Input: dimensioned drawing with shaded views. Units: mm. Origin: part minimum x, y, z. Give positions to 0.01 mm unless a question says otherwise; leave off trailing zeros. Write each loop counter-clockwise with the first axis right and the second up, starting at its lowest first coordinate (ties: lowest second). Pieces come first, ordered by that corner, then holes. Notation, with made-up numbers: (85, 56) -> (117, 56) arc R22 cw to (117, 68) -> close; hole circle Ø5 at (-36.75, 42). An arc over 180 degrees is marked (long way). Answer in a Markdown table with one row per item. Add a question column.
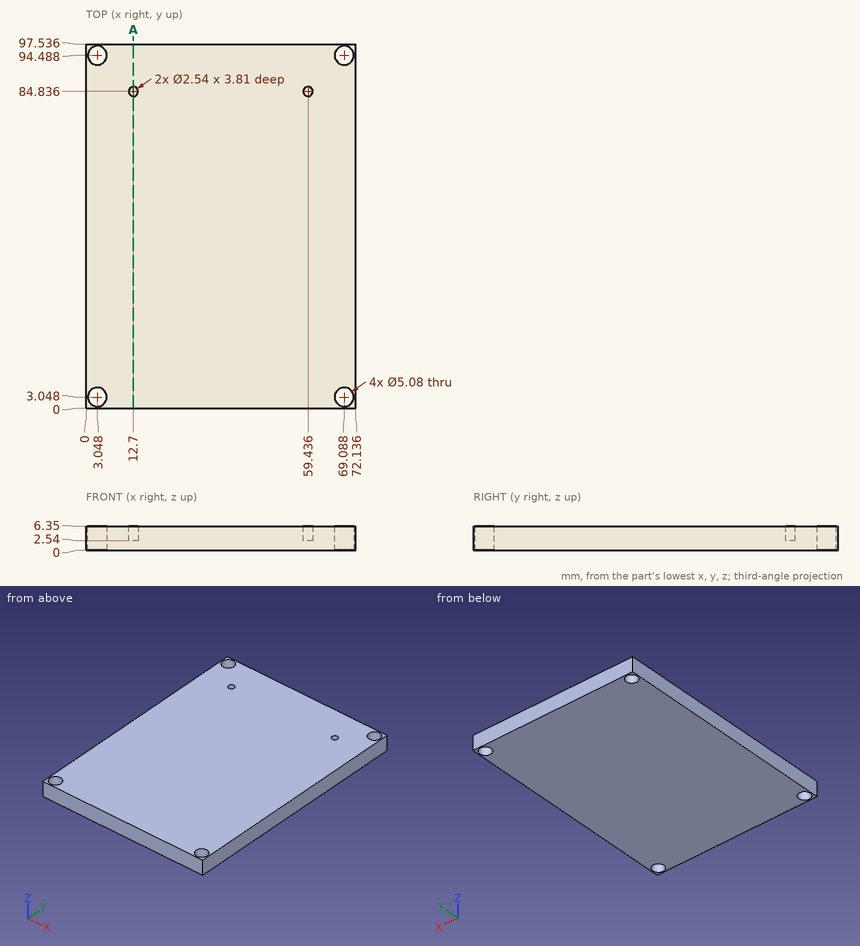
Q1. Line query: probe 1 along Y at (x, z) = (69, 5.25); probe 2 along X at (y, z) = (92.5, 5); probe 3 along Y at (x, z) = (12.7, 4.85). Output: solid intervals per line, ascending. Write a range as from..to.
Q2. Section A-A on x = 12.7. Return loops of the section in (y, z), and give its area (3 significant figures).
Q3. Contact query for flat-ended pins moving along their axis: pin 1 Ø3 at (x, y) = (3.048, 3.048) entering from -Z; pin 2 Ø0.8 at (x, y) = (59, 84.5) entering from +Z. Output: stop coordinate, or through.
Checks:
| question | item | result |
|---|---|---|
| 1 | probe 1 | 0..0.51, 5.59..91.95, 97.03..97.54 |
| 1 | probe 2 | 0..1.47, 4.63..67.51, 70.67..72.14 |
| 1 | probe 3 | 0..83.57, 86.11..97.54 |
| 2 | outline | (0, 0) -> (97.54, 0) -> (97.54, 6.35) -> (86.11, 6.35) -> (86.11, 2.54) -> (83.57, 2.54) -> (83.57, 6.35) -> (0, 6.35) -> close |
| 2 | area | 610 mm^2 |
| 3 | pin 1 | through |
| 3 | pin 2 | z = 2.54 |
